For this review, take the finished solid that the model builds, in its own axes (mm). Face numbers are marked on the shaded views. A direction names the side the tool comes from. Round coordinates to 2 decimals unless told otherwise and drop trailing zeros. Write each loop counter-clockwise with the first axis right and the second up, starting at its lowest first coordinate (ties: lowest second). Pieces come first, ordered by that corner, then holes. Notation, with made-up numbers: M 8,35 L 37,35 A20 ccw 37,60 Z; hole C -9.75,39 d7. An arc over 180 degrees is marked long. Write each question's results on one line, items separated by ' | '. Start each with the question number.
```python
from build123d import *

# Parameters (mm, degrees)
SKETCH_R      = 7
PAD_DEPTH     = 2
SKETCH001_R   = 6
PAD001_DEPTH  = 12
SKETCH002_W   = 0.5
SKETCH002_H   = 3
SKETCH002_W_2 = 3
SKETCH002_H_2 = 0.5
PAD002_DEPTH  = 5
SKETCH003_R   = 3
POCKET_DEPTH  = 10
SKETCH004_R   = 1
PAD003_DEPTH  = 8


with BuildPart() as part:
    # Sketch → Pad (new body)
    with BuildSketch(Plane.XY):
        Circle(SKETCH_R)
    extrude(amount=PAD_DEPTH)

    # Sketch001 (on Face3 of Pad) → Pad001 (join)
    with BuildSketch(Plane.XY.offset(2)):
        Circle(SKETCH001_R)
    extrude(amount=PAD001_DEPTH)

    # Sketch002 (on Face5 of Pad001) → Pad002 (join)
    with BuildSketch(Plane.XY.offset(14)):
        with Locations((-1.25, 3)):
            Rectangle(SKETCH002_W, SKETCH002_H)
        with Locations((-3.25, -2.5)):
            Rectangle(SKETCH002_W, SKETCH002_H)
        with Locations((2, -4.25)):
            Rectangle(SKETCH002_W_2, SKETCH002_H_2)
    extrude(amount=PAD002_DEPTH)

    # Sketch003 (on Face2 of Pad002) → Pocket (cut)
    with BuildSketch(Plane(origin=(0, 0, 0), x_dir=(1, 0, 0), z_dir=(0, 0, -1))):
        with Locations((3, 0)):
            Circle(SKETCH003_R)
    extrude(amount=-POCKET_DEPTH, mode=Mode.SUBTRACT)

    # Sketch004 (on Face6 of Pocket) → Pad003 (join)
    with BuildSketch(Plane(origin=(0, 0, 10), x_dir=(1, 0, 0), z_dir=(0, 0, -1))):
        with Locations((3, 0)):
            Circle(SKETCH004_R)
    extrude(amount=PAD003_DEPTH)


solid = part.part
```
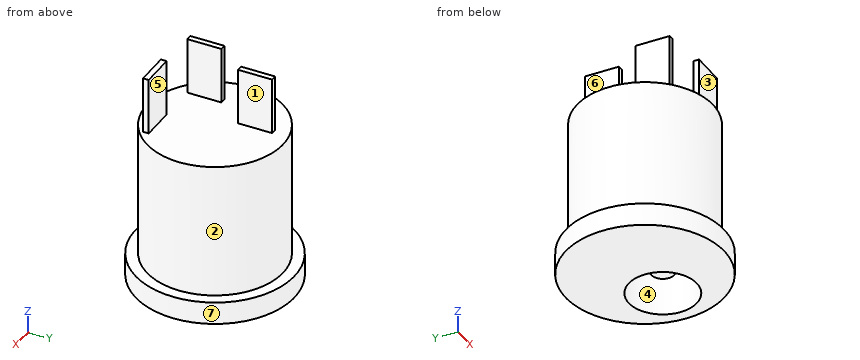
Item 1: For the marked faces 1, 2 and 3, list the 3-axis set-ups (+Z, -Z, +X, -X, +Y, -Y) from which the entire face can be reached by the end or side of a thin tool; tool diameter is ignored.
Item 2: For probe 1 along Z at (x, y) = (-5.5, -3.5); probe 2 along Z at (x, y) = (-1, -2.5); probe 3 along X at (y, z) = (-2.5, 15.25), list the stretches that pass through material, from the lowest coordinate up.
Item 3: We need section C-C on z = 1.75. State the section outline as (x, y) points, then the cut area to 3 significant figures.
Item 4: We need section B-B on y = 1.25. State the section outline as (x, z) points, then the cut area to 3 significant figures.
Item 5: We need section A-A on x = 3. State the section outline as (y, z) points, then the cut area to 3 significant figures.
Item 6: We need section D-D on x = -4.5. State the section outline as (y, z) points.
Item 7: Insertion check: P1, Ø0.6, axis at x = 3, y = -0.5, coming from the -Z side; P2, Ø1.5, axis at x = 2.5, z = 17.5, coming from the -Y side; P3, Ø0.6, axis at x = -1, z = 16, coming from the -Y side; P4, Ø1.5, axis at x = -5.5, y = -2.5, coming from the -Z side. Each pin has a flat end and moves straight along its axis. Give the tip position at first contact, or say it passes through.
Item 8: Mouldability with a two-part tool opening along Y and no side actions: class the marked faces 4, 5, 6 and 7 as pulls with the +Y half, pulls with the -Y half, needs draft (parallel to the pull), parting line crosses it, or undercut.
Numbers:
1) face 1: +Z, +X, +Y, -Y | face 2: +Z | face 3: +Z, +X, -X, -Y
2) probe 1: z = 0 to 2 | probe 2: z = 0 to 14 | probe 3: x = -3.5 to -3
3) outline: C 0,0 d14; hole C 3,0 d6 | area: 126 mm^2
4) outline: M -6.89,0 L 0.27,0 L 0.27,10 L 5.73,10 L 5.73,0 L 6.89,0 L 6.89,2 L 5.87,2 L 5.87,14 L -5.87,14 L -5.87,2 L -6.89,2 Z | area: 114 mm^2
5) outline: M -6.32,0 L -3,0 L -3,10 L -1,10 L -1,2 L 1,2 L 1,10 L 3,10 L 3,0 L 6.32,0 L 6.32,2 L 5.2,2 L 5.2,14 L -4,14 L -4,19 L -4.5,19 L -4.5,14 L -5.2,14 L -5.2,2 L -6.32,2 Z | area: 109 mm^2
6) outline: M -5.36,0 L 5.36,0 L 5.36,2 L 3.97,2 L 3.97,14 L -3.97,14 L -3.97,2 L -5.36,2 Z
7) P1: stops at z = 2 | P2: stops at y = -4.5 | P3: stops at y = 1.5 | P4: stops at z = 0
8) face 4: undercut | face 5: pulls with the +Y half | face 6: needs draft | face 7: parting line crosses it
